Autodesk Inventor part; units mm, degrees
ref_plane "Work Plane1" through (5, 0.5, -14) normal (0, 0, -1) x (-1, 0, 0)
ref_plane "YZ Plane" through (0, 0, 0) normal (1, 0, 0) x (0, 1, 0)
ref_plane "XZ Plane" through (0, 0, 0) normal (0, 1, 0) x (-1, 0, 0)
sketch "Sketch1" plane through (0, 0, 0) normal (0, 1, 0) x (-1, 0, 0)
  line L0 (0, 0) -> (-30, 0)
  line L1 (-30, 0) -> (-30, -20)
  line L2 (-30, -20) -> (0, -20)
  line L3 (0, -20) -> (0, 0)
  dimension "d0" = 30
  dimension "d1" = 20
extrude "Plate1" add sketch "Sketch1" along normal blind 0.5
sketch "Sketch2" plane through (0, 0.5, 0) normal (0, 1, 0) x (1, 0, 0)
  line L0 (5, 14) -> (25, 14)
  line L1 (25, 14) -> (25, 6)
  line L2 (25, 6) -> (5, 6)
  line L3 (5, 6) -> (5, 14)
  line L4 (5, 14) -> (25, 6) construction
  line L5 (25, 14) -> (5, 6) construction
  line L6 (0, 0) -> (0, 20)
  line L7 (30, 0) -> (0, 0)
  point P0 (15, 10)
  dimension "d3" = 15
  dimension "d4" = 10
  dimension "d5" = 20
  dimension "Width" = 8
extrude "Extrusion1" cut sketch "Sketch2" against normal blind 0.5
ref_plane "Work Plane1" through (5, 0.5, -14) normal (0, 0, -1) x (-1, 0, 0)
sketch "Sketch3" plane through (5, 0.5, -14) normal (0, 0, -1) x (-1, 0, 0)
  line L0 (-20, 0) -> (0, 0)
  arc A0 (0, 0) -> (-2, -2) centre (0, -2) ccw
  arc A1 (-4, -4) -> (-2, -2) centre (-4, -2) ccw
  line L1 (-4, -4) -> (-16, -4)
  arc A2 (-18, -2) -> (-16, -4) centre (-16, -2) ccw
  arc A3 (-18, -2) -> (-20, 0) centre (-20, -2) ccw
  line L2 (0, 0) -> (-20, 0)
  arc A4 (-18.5, -2) -> (-20, -0.5) centre (-20, -2) ccw
  arc A5 (-18.5, -2) -> (-16, -4.5) centre (-16, -2) ccw
  line L3 (-16, -4.5) -> (-4, -4.5)
  arc A6 (-4, -4.5) -> (-1.5, -2) centre (-4, -2) ccw
  arc A7 (0, -0.5) -> (-1.5, -2) centre (0, -2) ccw
  line L4 (-20, -0.5) -> (-20, 0)
  line L5 (0, -0.5) -> (0, 0)
  point P0 (5, -0.5)
  dimension "d9" = 2
  dimension "d10" = 0.5
extrude "Extrusion2" add sketch "Sketch3" against normal blind 8 contours A3 A2 L1 A1 A0 L5 A7 A6 L3 A5 A4 L4
sketch "Sketch4" plane through (9, -3.5, -14) normal (0, 1, 0) x (1, 0, 0)
  circle A0 centre (6, -4) radius 2
  point P0 (-9, -14)
  dimension "d13" = 4
extrude "Extrusion3" cut sketch "Sketch4" against normal blind 0.5
equation "\"d7\" = Thickness"
equation "\"d10\" = Thickness"
equation "\"d11\" = Width"
equation "\"d14\" = Thickness"
equation "\"d2\" = Thickness"
equation "\"BendRadius\" = Thickness"
equation "\"BendReliefWidth\" = Thickness"
equation "\"BendReliefDepth\" = 0.5 * Thickness"
equation "\"CornerReliefSize\" = 4 * Thickness"
equation "\"MinimumRemnant\" = 2 * Thickness"
equation "\"TransitionRadius\" = BendRadius"
equation "\"JacobiRadiusSize\" = BendRadius"
equation "\"GapSize\" = Thickness"
properties part number "CE-4.1.3"
The model under review builds one solid part; all positions refer to its coordinate system, in mm. A direction names the side the tool comes from. Coordinates: 2 decimals unless noted, no trailing zeros. Write each loop counter-clockwise with the first axis right and the second up, starting at its lowest first coordinate (ties: lowest second). Pieces come first, ordered by that corner, then holes. Notation, with made-up numbers: (-37, 9) -> (17, 9) arc R24 cw to (17, 46) -> close; hole circle Ø10 at (-30, 41.25). An arc over 180 degrees is marked (long way). One line per item, written item: value. Start each with the question number.
Q1. Clearance check with flat-ended pins moving along their axes: P1, Ø1, axis at y = -2.5, z = -10, coming from the +X side; P2, Ø1, axis at x = 10.5, z = -3, coming from the -Y side; P3, Ø4, axis at x = 14.5, z = -11, coming from the +Y side; P4, Ø2, axis at x = 10, y = -0.5, coming from the -Z side. State where each tip first meets the part, or that it passes through.
Q2. To check wall thickness, follow probe 1 along Z at (x, y) = (15, -3.7); probe 2 along Y at (x, z) = (20, -19); probe 3 along Y at (x, z) = (15, -7). State the ranges of each line that lie inside material, in increasing order.
Q3. Add section D-D, the plane z = -6.5. Give the boundary of the cut face in (x, y), then the cut area to 3 significant figures.
Q4. For faces 4 (the face through (16, -3.5, -12)), 5 (the face through (7, -3, -10)), list the 3-axis set-ups (+Z, -Z, +X, -X, +Y, -Y) from which the entire face can be reached by the end or side of a thin tool; tool diameter is ignored.
Q5. Add section C-C, the plane y = -2.35. Give the boundary of the cut face in (x, z), then the cut area to 3 significant figures.
Q6. The part is to be moulded in two halves that separate along Z. For faces 1 (the face through (15, -3.8, -14)), 2 (the face through (13.526, -3.746, -11.352)), 3 (the face through (15, -3.8, -6)), say which applies: +Z half, -Z half, draft (parallel to the pull), parting line (faces both ways), or undercut.
Q7. Add section B-B, the plane z = -10. Give the boundary of the cut face in (x, y), then the cut area to 3 significant figures.
Q8. Add section A-A, the plane x = 15. Give the boundary of the cut face in (y, z), then the cut area to 3 significant figures.
Response:
1. P1: x = 23.45
1. P2: y = 0
1. P3: y = -3.5
1. P4: z = -20
2. probe 1: -14 to -12, -8 to -6
2. probe 2: 0 to 0.5
2. probe 3: -4 to -3.5
3. outline: (0, 0) -> (5, 0) arc R1.5 cw to (6.5, -1.5) arc R2.5 ccw to (9, -4) -> (21, -4) arc R2.5 ccw to (23.5, -1.5) arc R1.5 cw to (25, 0) -> (30, 0) -> (30, 0.5) -> (25, 0.5) arc R2 ccw to (23, -1.5) arc R2 cw to (21, -3.5) -> (9, -3.5) arc R2 cw to (7, -1.5) arc R2 ccw to (5, 0.5) -> (0, 0.5) -> close
3. area: 17.3 mm²
4. face 4: +Z, -Z, +Y
4. face 5: +Z, -Z, -X, -Y
5. outline: (6.65, -14) -> (7.19, -14) -> (7.19, -6) -> (6.65, -6) -> close; (22.81, -14) -> (23.35, -14) -> (23.35, -6) -> (22.81, -6) -> close
5. area: 8.65 mm²
6. face 1: -Z half
6. face 2: undercut
6. face 3: +Z half
7. outline: (0, 0) -> (5, 0) arc R1.5 cw to (6.5, -1.5) arc R2.5 ccw to (9, -4) -> (13, -4) -> (13, -3.5) -> (9, -3.5) arc R2 cw to (7, -1.5) arc R2 ccw to (5, 0.5) -> (0, 0.5) -> close; (17, -4) -> (21, -4) arc R2.5 ccw to (23.5, -1.5) arc R1.5 cw to (25, 0) -> (30, 0) -> (30, 0.5) -> (25, 0.5) arc R2 ccw to (23, -1.5) arc R2 cw to (21, -3.5) -> (17, -3.5) -> close
7. area: 15.3 mm²
8. outline: (-4, -14) -> (-3.5, -14) -> (-3.5, -12) -> (-4, -12) -> close; (-4, -8) -> (-3.5, -8) -> (-3.5, -6) -> (-4, -6) -> close; (0, -20) -> (0.5, -20) -> (0.5, -14) -> (0, -14) -> close; (0, -6) -> (0.5, -6) -> (0.5, 0) -> (0, 0) -> close
8. area: 8.00 mm²
